Input: part model. Units: mm. Frame: model coordinates. Face numbers are marked on the shaded views. A direction names the side the tool comes from. Coordinates: 2 decimals unless noted, no trailing zeros. Order: outer loops, then holes, each group sorted by start corner. A loop starts at its lowest first (then second) coordinate and runs counter-clockwise, first axis right, second up.
from build123d import *

# Parameters (mm, degrees)
BOSS_EXTRUDE1_DEPTH      = 39
CUT_EXTRUDE1_DEPTH       = 35.6
CUT_EXTRUDE1_DEPTH_BACK  = 35.6
SKETCH2_W                = 71.5
SKETCH2_H                = 71.5
CUT_EXTRUDE2_DEPTH       = 10
SKETCH5_W                = 68.2
SKETCH5_H                = 8.5
SKETCH5_H_2              = 7.95
SKETCH5_H_3              = 24.7
CUT_EXTRUDE3_DEPTH       = 3.1
CHAMFER1_SIZE            = 3.1
CHAMFER1_OF_MIRROR1_SIZE = 3.1
FILLET1_R                = 1


with BuildPart() as part:
    # Sketch1 → Boss-Extrude1 (new, symmetric)
    with BuildSketch(Plane.XY):
        Polygon((-78, 0), (0, 0), (0, 78), (-9, 78), (-9, 73), (-73, 9), (-78, 9), align=None)
    extrude(amount=BOSS_EXTRUDE1_DEPTH, both=True)

    # Sketch2 → Cut-Extrude1 (cut, two sides: drawn at the far end of the back side and taken through both)
    with BuildSketch(Plane.XY.offset(-CUT_EXTRUDE1_DEPTH_BACK)):
        with Locations((-42.25, 42.25)):
            Rectangle(SKETCH2_W, SKETCH2_H)
    extrude(amount=CUT_EXTRUDE1_DEPTH + CUT_EXTRUDE1_DEPTH_BACK, mode=Mode.SUBTRACT)

    # Sketch3 → Cut-Extrude2 (cut)
    with BuildSketch(Plane(origin=(0, 6.5, 0), x_dir=(1, 0, 0), z_dir=(0, 1, 0))):
        with BuildLine():
            Line((-27.25, -24.25), (-37.75, -24.25))
            ThreePointArc((-37.75, -24.25), (-42, -20), (-37.75, -15.75))
            Line((-37.75, -15.75), (-27.25, -15.75))
            ThreePointArc((-27.25, -15.75), (-23, -20), (-27.25, -24.25))
        make_face()
        with BuildLine():
            Line((-60.25, -15.75), (-58.25, -15.75))
            ThreePointArc((-58.25, -15.75), (-54, -20), (-58.25, -24.25))
            Line((-58.25, -24.25), (-60.25, -24.25))
            ThreePointArc((-60.25, -24.25), (-64.5, -20), (-60.25, -15.75))
        make_face()
        with BuildLine():
            Line((-27.25, 24.25), (-37.75, 24.25))
            ThreePointArc((-37.75, 24.25), (-42, 20), (-37.75, 15.75))
            Line((-37.75, 15.75), (-27.25, 15.75))
            ThreePointArc((-27.25, 15.75), (-23, 20), (-27.25, 24.25))
        make_face()
        with BuildLine():
            Line((-60.25, 15.75), (-58.25, 15.75))
            ThreePointArc((-58.25, 15.75), (-54, 20), (-58.25, 24.25))
            Line((-58.25, 24.25), (-60.25, 24.25))
            ThreePointArc((-60.25, 24.25), (-64.5, 20), (-60.25, 15.75))
        make_face()
    cut_extrude2 = extrude(amount=-CUT_EXTRUDE2_DEPTH, mode=Mode.SUBTRACT)

    # Sketch5 → Cut-Extrude3 (cut)
    with BuildSketch(Plane.XZ):
        with Locations((-37.5, 20)):
            Rectangle(SKETCH5_W, SKETCH5_H)
        with Locations((-37.5, 31.625)):
            Rectangle(SKETCH5_W, SKETCH5_H_2)
        with Locations((-37.5, 0)):
            Rectangle(SKETCH5_W, SKETCH5_H_3)
        with Locations((-37.5, -31.625)):
            Rectangle(SKETCH5_W, SKETCH5_H_2)
        with Locations((-37.5, -20)):
            Rectangle(SKETCH5_W, SKETCH5_H)
    cut_extrude3 = extrude(amount=-CUT_EXTRUDE3_DEPTH, mode=Mode.SUBTRACT)

    # Chamfer1
    chamfer1_edges = [part.edges().sort_by_distance(p)[0] for p in [
        (-3.4, 3.1, 31.625),
        (-3.4, 3.1, 20),
        (-3.4, 3.1, 0),
        (-3.4, 3.1, -20),
        (-3.4, 3.1, -31.625),
    ]]
    chamfer(chamfer1_edges, length=CHAMFER1_SIZE - 0.0001)  # a hair under: the kernel refuses the full size

    # Mirror1: Cut-Extrude2, Cut-Extrude3 across plane
    add(cut_extrude2.mirror(Plane(origin=(0, 0, 0), x_dir=(0, 0, 1), z_dir=(-0.7071067811865474, -0.7071067811865477, 0))), mode=Mode.SUBTRACT)
    add(cut_extrude3.mirror(Plane(origin=(0, 0, 0), x_dir=(0, 0, 1), z_dir=(-0.7071067811865474, -0.7071067811865477, 0))), mode=Mode.SUBTRACT)

    # Chamfer1 of Mirror1
    chamfer1_of_mirror1_edges = [part.edges().sort_by_distance(p)[0] for p in [
        (-3.1, 3.4, 31.625),
        (-3.1, 3.4, 20),
        (-3.1, 3.4, 0),
        (-3.1, 3.4, -20),
        (-3.1, 3.4, -31.625),
    ]]
    chamfer(chamfer1_of_mirror1_edges, length=CHAMFER1_OF_MIRROR1_SIZE - 0.0001)  # a hair under: the kernel refuses the full size

    # Fillet1
    fillet1_edges = [part.edges().sort_by_distance(p)[0] for p in [
        (-78, 9, 37.3),
        (-73, 9, 37.3),
        (-9, 73, 37.3),
        (-9, 78, 37.3),
        (-78, 9, -37.3),
        (-73, 9, -37.3),
        (-9, 73, -37.3),
        (-9, 78, -37.3),
    ]]
    fillet(fillet1_edges, radius=FILLET1_R)


solid = part.part
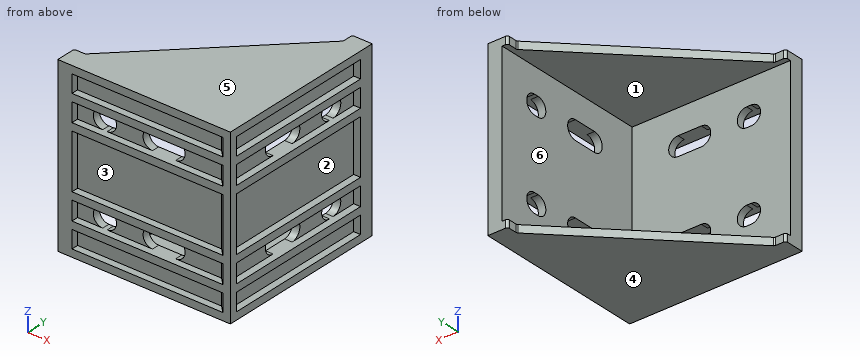
Item 1: Pin query (flat end, axial travel): pin 1 Ø4 at (x, z) = (-41.5, -20.5) entering from +Y; pin 2 Ø5 at (y, z) = (60.5, 3) entering from -X; pin 3 Ø4 at (x, z) = (-68, 22) entering from -Y. Return the tip coordinate at first contact, or that it passes through.
Response values:
pin 1: stops at y = 6.5
pin 2: stops at x = -6.5
pin 3: stops at y = 3.1
Item 2: Cut plane A-A on z = 20. Count the separate pieces of the cut face and the enclosed holes in it, then the cut area to 3 significant figures.
Response values:
separate pieces: 5
enclosed holes: 0
area: 358 mm2
Item 3: Access query for the marked faces 1, 2 and 3. Directions: +Z, -Z, +X, -X, +Y, -Y. A direction counts if a zero-diameter tool reaches every point of the face in a straight line with its end or side. Return the directions, or none.
Response values:
face 1: -X, +Y
face 2: +X
face 3: -Y
Item 4: Cut plane C-C on y = 48.5. Return loops of the section in (x, z), then the cut area to 3 significant figures.
Response values:
outline: (-33.5, -39) - (0, -39) - (0, -35.6) - (-3.1, -35.6) - (-3.1, -27.65) - (0, -27.65) - (0, -24.25) - (-3.1, -24.25) - (-3.1, -15.75) - (0, -15.75) - (0, -12.35) - (-3.1, -12.35) - (-3.1, 12.35) - (0, 12.35) - (0, 15.75) - (-3.1, 15.75) - (-3.1, 24.25) - (0, 24.25) - (0, 27.65) - (-3.1, 27.65) - (-3.1, 35.6) - (0, 35.6) - (0, 39) - (-33.5, 39) - (-33.5, 35.6) - (-6.5, 35.6) - (-6.5, -35.6) - (-33.5, -35.6) - close
area: 512 mm2
Item 5: Draft query along Z for the marked faces 4, 5 and 6. Return one class per face: pulls with the +Z half, pulls with the -Z half, needs draft (parallel to the pull), parting line crosses it, or undercut.
Response values:
face 4: pulls with the -Z half
face 5: pulls with the +Z half
face 6: undercut
Item 6: Ray query, probe 1 along Z at (x, y) = (-9.5, 3); probe 2 along Z at (x, y) = (-29, 34.5); probe 3 along Y at (x, z) = (-21.5, -1.5). Return the intervals inside material, ascending.
Response values:
probe 1: z = -39 to -35.6, -27.65 to -24.25, -15.75 to -12.35, 12.35 to 15.75, 24.25 to 27.65, 35.6 to 39
probe 2: z = -39 to -35.6, 35.6 to 39
probe 3: y = 3.1 to 6.5
Item 7: Cut plane B-B on x = -70. Return loops of the section in (y, z).
Response values:
outline: (0, -39) - (12, -39) - (12, -35.6) - (6.5, -35.6) - (6.5, 35.6) - (12, 35.6) - (12, 39) - (0, 39) - (0, 35.6) - (3.1, 35.6) - (3.1, 27.65) - (0, 27.65) - (0, 24.25) - (3.1, 24.25) - (3.1, 15.75) - (0, 15.75) - (0, 12.35) - (3.1, 12.35) - (3.1, -12.35) - (0, -12.35) - (0, -15.75) - (3.1, -15.75) - (3.1, -24.25) - (0, -24.25) - (0, -27.65) - (3.1, -27.65) - (3.1, -35.6) - (0, -35.6) - close
